Autodesk Inventor part; units mm, degrees
ref_plane "to_bolt_XY" through (10, 15, 12.5) normal (0, 0, 1) x (1, 0, 0)
ref_plane "to_bolt_YZ" through (10, 15, 12.5) normal (1, 0, 0) x (0, 1, 0)
ref_plane "to_bolt_ZX" through (10, 15, 12.5) normal (0, 1, 0) x (0, 0, 1)
sketch "_____8" plane through (0, 0, 0) normal (1, 0, 0) x (0, 0, -1)
  line L0 (-30, 5.1358) -> (-30, -5.1358)
  arc A0 (-30, -5.1358) -> (-28.7299, -6.9979) centre (-28, -5.1358) ccw
  line L1 (-28.7299, -6.9979) -> (-6.204, -15.8275)
  arc A1 (-6.204, -15.8275) -> (6.204, -15.8275) centre (0, 0) ccw
  line L2 (6.204, -15.8275) -> (28.7299, -6.9979)
  arc A2 (28.7299, -6.9979) -> (30, -5.1358) centre (28, -5.1358) ccw
  line L3 (30, -5.1358) -> (30, 5.1358)
  arc A3 (30, 5.1358) -> (28.7299, 6.9979) centre (28, 5.1358) ccw
  line L4 (28.7299, 6.9979) -> (18.8506, 10.8703)
  arc A4 (12.5986, 18.7801) -> (18.8506, 10.8703) centre (22.5, 20.1806) ccw
  arc A5 (12.5986, 18.7801) -> (10.6183, 20.5) centre (10.6183, 18.5) ccw
  line L5 (10.6183, 20.5) -> (-10.6183, 20.5)
  arc A6 (-10.6183, 20.5) -> (-12.5986, 18.7801) centre (-10.6183, 18.5) ccw
  arc A7 (-18.8506, 10.8703) -> (-12.5986, 18.7801) centre (-22.5, 20.1806) ccw
  line L6 (-18.8506, 10.8703) -> (-28.7299, 6.9979)
  arc A8 (-28.7299, 6.9979) -> (-30, 5.1358) centre (-28, 5.1358) ccw
extrude "Extrusion1" add sketch "_____8" along normal blind 20
sketch "_____2" plane through (0, 0, 0) normal (1, 0, 0) x (0, 0, -1)
  line L0 (-1, 37.5) -> (-1, -12)
  line L1 (-1, -12) -> (1, -12)
  line L2 (1, -12) -> (1, 37.5)
  line L3 (1, 37.5) -> (-1, 37.5)
extrude "Extrusion2" cut sketch "_____2" along normal blind 20
sketch "_____3" plane through (0, 0, 0) normal (0, 0, 1) x (1, 0, 0)
  line L0 (20, 0) -> (0, 0)
  line L1 (0, 0) -> (0, 10.8)
  line L2 (0, 10.8) -> (0.8, 10)
  line L3 (0.8, 10) -> (19.2, 10)
  line L4 (19.2, 10) -> (20, 10.8)
  line L5 (20, 10.8) -> (20, 0)
  line L6 (20, 0) -> (0, 0)
revolve "Revolution1" cut sketch "_____3" angle 360 about axis through (20, 0, 0) along (1, 0, 0)
sketch "_____4" plane through (0, 0, 24) normal (0, 0, 1) x (1, 0, 0)
  line L0 (20, 0) -> (0, 0)
  line L1 (0, 0) -> (0, 4)
  line L2 (0, 4) -> (0.5, 3.5)
  line L3 (0.5, 3.5) -> (19.5, 3.5)
  line L4 (19.5, 3.5) -> (20, 4)
  line L5 (20, 4) -> (20, 0)
  line L6 (20, 0) -> (0, 0)
revolve "Revolution2" cut sketch "_____4" angle 360 about axis through (20, 0, 24) along (1, 0, 0)
pattern_linear "Rectangular Pattern1" count 2 spacing 48 along (0, 0, -1) of "Revolution2"
sketch "Sketch5" plane through (0, 20.5, -1) normal (0, 0, 1) x (1, 0, 0)
  point P0 (10, -5.5)
hole "Hole1" at (10, 15, -1) direction (0, 0, -1) diameter 4.134 depth 16.5 countersink diameter 5 countersink angle 90
sketch "Sketch6" plane through (20, 20.5, 1) normal (0, 0, -1) x (-1, 0, 0)
  point P0 (10, -5.5)
hole "Hole2" at (10, 15, 1) direction (0, 0, 1) diameter 5.5 depth 25
sketch "_____9" plane through (0, 0, 12.5) normal (0, 0, 1) x (1, 0, 0)
  line L0 (5, 33.75) -> (5, 15)
  arc A0 (5, 15) -> (15, 15) centre (10, 15) ccw
  line L1 (15, 15) -> (15, 33.75)
  line L2 (15, 33.75) -> (5, 33.75)
extrude "Extrusion3" cut sketch "_____9" along normal blind 20
ref_plane "to_bolt_XY" through (10, 15, 12.5) normal (0, 0, 1) x (1, 0, 0)
ref_plane "to_bolt_YZ" through (10, 15, 12.5) normal (1, 0, 0) x (0, 1, 0)
ref_plane "to_bolt_ZX" through (10, 15, 12.5) normal (0, 1, 0) x (0, 0, 1)
properties part number "C-SHFMQ20_b"
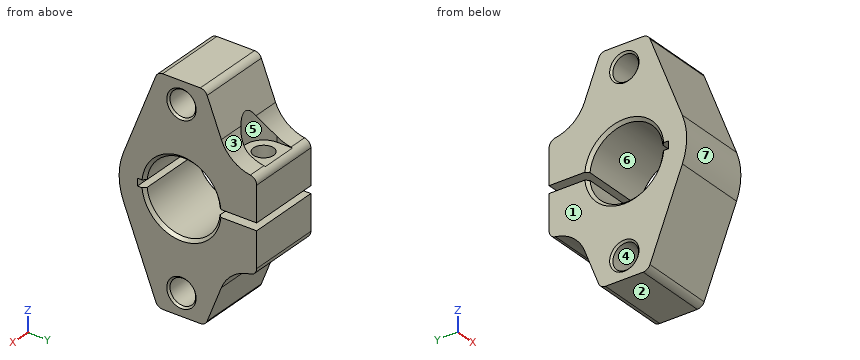
The model under review builds one solid part; all positions refer to its coordinate system, in mm. Face numbers are marked on the shaded views. A direction names the side the tool comes from. Round coordinates to 2 decimals unless told otherwise and drop trailing zeros. Write each loop counter-clockwise with the first axis right and the second up, starting at its lowest first coordinate (ties: lowest second). Pieces come first, ordered by that corner, then holes. Notation, with made-up numbers: M 62,-35 L 73,-35 A7 cw 73,-27 Z; hole C -1,23 d3. An arc over 180 degrees is marked long. Use CSV: the item, a comma, the result in double quotes. Start each with the question number.
(1) Clearance check with flat-ended pins moving along their axes: P1, Ø4, axis at y = 0, z = 24, coming from the -X side; P2, Ø6.5, axis at x = 10, y = 15, coming from the +Z side; P3, Ø3, axis at x = 8, y = 13, coming from the -Z side; P4, Ø1, axis at x = 16.5, z = -23.5, coming from the -Y side. State where each tip first meets the part, or that it passes through.
(2) We need section B-B, the plane z = -24. State the section outline as (x, y) points.
(3) We need section A-A, the plane x = 3. State the section outline as (y, z) points, then the cut area to 3 significant figures.
(4) Tool access review of the marked faces 5, 6 and 7: name each direction out of +Z, -Z, +X, -X, +Y, -Y from which nothing blocks a thin tool from reaching the whole face with its end or side.
(5) We need section C-C, the plane x = 10. State how many separate pieces and enclosed holes the cut face has, then the cut area to 3 significant figures.
(6) For line 1 along Z through (x, y) = (15.5, 0); line 2 along X through (y, z) = (15, -9); line 3 along Z through (x, y) = (10.5, 1), list the stretches that pass through material, from the lowest coordinate up.
(7) The part is to be moulded in two halves that separate along Z. For the marked faces 1, 2, 3 and 4, say which applies: +Z half, -Z half, draft (parallel to the pull), parting line (faces both ways), or undercut.
Findings:
1,P1,"through"
1,P2,"z = 12.5"
1,P3,"z = -17.54"
1,P4,"y = -9.24"
2,outline,"M 0,-8.85 L 20,-8.85 L 20,-4 L 19.5,-3.5 L 0.5,-3.5 L 0,-4 Z; M 0,4 L 0.5,3.5 L 19.5,3.5 L 20,4 L 20,8.85 L 0,8.85 Z"
3,outline,"M -15.83,-6.2 L -7,-28.73 A2 ccw -5.14,-30 L 5.14,-30 A2 ccw 7,-28.73 L 10.87,-18.85 A10 cw 18.78,-12.6 A2 ccw 20.5,-10.62 L 20.5,-1 L 9.95,-1 A10 cw -9.95,-1 L -12,-1 L -12,1 L -9.95,1 A10 cw 9.95,1 L 20.5,1 L 20.5,10.62 A2 ccw 18.78,12.6 A10 cw 10.87,18.85 L 7,28.73 A2 ccw 5.14,30 L -5.14,30 A2 ccw -7,28.73 L -15.83,6.2 A17 ccw Z; hole C 0,-24 d7; hole C 0,24 d7"
3,area,"1,200 mm^2"
4,face 5,"+Z, +Y"
4,face 6,"+X, -X"
4,face 7,"+X, -X, -Y"
5,separate pieces,"3"
5,enclosed holes,"2"
5,area,"1,060 mm^2"
6,line 1,"-30 to -27.5, -20.5 to -10, 10 to 20.5, 27.5 to 30"
6,line 2,"0 to 7.93, 12.07 to 20"
6,line 3,"-30 to -27.35, -20.65 to -9.95, 9.95 to 20.65, 27.35 to 30"
7,face 1,"draft"
7,face 2,"-Z half"
7,face 3,"+Z half"
7,face 4,"undercut"
